Work out the finished part from the listing and answer in its coordinate system (mm). Face numbers are marked on the shaded views. A direction names the side the tool comes from. Give positions to 0.01 mm unless a question says otherwise; leave off trailing zeros. Loops run counter-clockwise (first coordinate to the right, second up) from the corner with the lowest first, then second, coordinate; pieces in that order, holes last. Notation, with made-up numbers: M 76,-16 L 87,-16 A28 cw 87,5 Z; hole C 83.5,63.5 d8. An arc over 180 degrees is marked long. Answer as a JSON object with one key per item and string values. Group by question number.
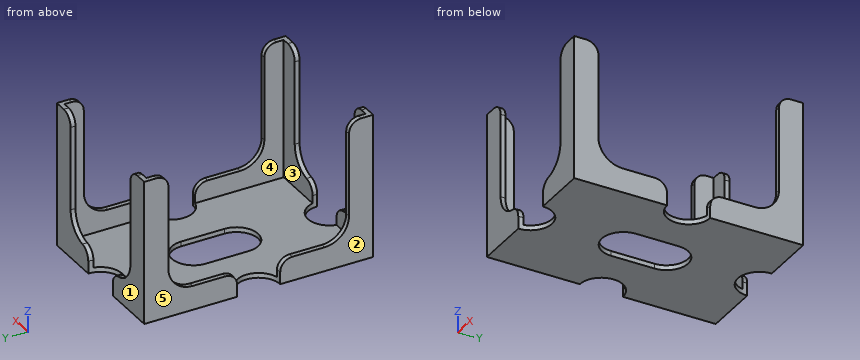
```python
from build123d import *

# Parameters (mm, degrees)
SKETCH008_W          = 50.7
SKETCH008_H          = 75.7
PAD002_DEPTH         = 47.6
THICKNESS002_T       = -1.6
POCKET004_DEPTH      = 37.851
POCKET004_DEPTH_BACK = 37.851
POCKET003_DEPTH      = 25.351
POCKET003_DEPTH_BACK = 25.351
SKETCH006_R          = 7.125
POCKET005_DEPTH      = 0.001
POCKET005_DEPTH_BACK = 47.601
FILLET001_R          = 4


with BuildPart() as part:
    # Sketch008 → Pad002 (new body)
    with BuildSketch(Plane.XY):
        Rectangle(SKETCH008_W, SKETCH008_H)
    extrude(amount=PAD002_DEPTH)

    # Thickness002
    thickness002_openings = [part.faces().sort_by_distance(p)[0] for p in [
        (0, 0, 47.6),
    ]]
    offset(amount=THICKNESS002_T, openings=thickness002_openings, kind=Kind.INTERSECTION)

    # Sketch007 → Pocket004 (cut, two sides)
    with BuildSketch(Plane.XZ) as pocket004_sk:
        with BuildLine():
            Line((-17.35, 47.6), (17.35, 47.6))
            Line((17.35, 47.6), (17.35, 16))
            ThreePointArc((9.35, 8), (15.006854, 10.343146), (17.35, 16))
            Line((9.35, 8), (-9.35, 8))
            ThreePointArc((-17.35, 16), (-15.006854, 10.343146), (-9.35, 8))
            Line((-17.35, 16), (-17.35, 47.6))
        make_face()
    extrude(amount=-POCKET004_DEPTH, mode=Mode.SUBTRACT)
    extrude(pocket004_sk.sketch, amount=POCKET004_DEPTH_BACK, mode=Mode.SUBTRACT)

    # Sketch005 → Pocket003 (cut, two sides)
    with BuildSketch(Plane.YZ) as pocket003_sk:
        with BuildLine():
            Line((-29.85, 47.6), (29.85, 47.6))
            Line((29.85, 47.6), (29.85, 16))
            ThreePointArc((21.85, 8), (27.506854, 10.343146), (29.85, 16))
            Line((21.85, 8), (-21.85, 8))
            ThreePointArc((-29.85, 16), (-27.506854, 10.343146), (-21.85, 8))
            Line((-29.85, 16), (-29.85, 47.6))
        make_face()
    extrude(amount=-POCKET003_DEPTH, mode=Mode.SUBTRACT)
    extrude(pocket003_sk.sketch, amount=POCKET003_DEPTH_BACK, mode=Mode.SUBTRACT)

    # Sketch006 → Pocket005 (cut, two sides)
    with BuildSketch(Plane.XY) as pocket005_sk:
        with Locations((0, 37.85)):
            Circle(SKETCH006_R)
        with Locations((0, -37.85)):
            Circle(SKETCH006_R)
        with Locations((25.35, 0)):
            Circle(SKETCH006_R)
        with Locations((-25.35, 0)):
            Circle(SKETCH006_R)
        with BuildLine():
            ThreePointArc((7.125, 7.125), (0, 14.25), (-7.125, 7.125))
            Line((-7.125, 7.125), (-7.125, -7.125))
            ThreePointArc((-7.125, -7.125), (0, -14.25), (7.125, -7.125))
            Line((7.125, 7.125), (7.125, -7.125))
        make_face()
    extrude(amount=-POCKET005_DEPTH, mode=Mode.SUBTRACT)
    extrude(pocket005_sk.sketch, amount=POCKET005_DEPTH_BACK, mode=Mode.SUBTRACT)

    # Fillet001
    fillet001_edges = [part.edges().sort_by_distance(p)[0] for p in [
        (24.544843, -7.079361, 8),
        (24.544843, 7.079361, 8),
        (24.55, 29.85, 47.6),
        (17.35, 37.05, 47.6),
        (7.079361, 37.044843, 8),
        (-7.079361, 37.044843, 8),
        (-17.35, 37.05, 47.6),
        (-24.55, 29.85, 47.6),
        (-24.544843, 7.079361, 8),
        (-24.544843, -7.079361, 8),
        (-24.55, -29.85, 47.6),
        (-17.35, -37.05, 47.6),
        (-7.079361, -37.044843, 8),
        (7.079361, -37.044843, 8),
        (17.35, -37.05, 47.6),
        (24.55, -29.85, 47.6),
    ]]
    fillet(fillet001_edges, radius=FILLET001_R)


solid = part.part
```
Item 1: A cutting plane is placed at D-D (y = 29). Determine the outline of the cut face in (x, z), and give its area (3 significant figures).
Item 2: A cutting plane is placed at B-B (x = 0). Determine the outline of the cut face in (y, z) (3 decimals), and give its area (3 significant figures).
Item 3: A cutting plane is placed at C-C (z = 29). Determine the outline of the cut face in (x, y), and give its area (3 significant figures).
Item 4: A cutting plane is placed at A-A (y = 0). Determine the outline of the cut face in (x, z) (3 decimals).
Item 5: Find the intervals of material crossed by probe 1 along Y at (x, z) = (19, 36); probe 2 along X at (y, z) = (-34, 20.5), in increasing order. Write a range as [from, to].
Item 6: For a pull along X with two mould halves and no side action, classify the marked faces 1, 2 and 3 as pulls with the +X half, pulls with the -X half, needs draft (parallel to the pull), parting line crosses it, or undercut.
Item 7: A tool of negligible diameter and unlimited length cuts with its end or side. For the marked faces 4 and 5, from which of +Z, -Z, +X, -X, +Y, -Y can it reach the whole face along a straight path? Write none if from no direction.
Item 8: Given pin 1 Ø1.8 at (x, y) = (-24.5, -17) entering from +Z; pin 2 Ø1.3 at (y, z) = (1.5, 1) entering from -X; pin 3 Ø4 at (x, y) = (-7.5, 26) entering from +Z; pin 4 Ø5 at (y, z) = (-26.5, 10) entering from +X, each flat-ended and moving along its own axis, determine where each tip first touches the part or whether it passes through.
The answers:
{
 "1": {"outline": "M -25.35,0 L 25.35,0 L 25.35,12.41 L 23.75,12.41 L 23.75,1.6 L -23.75,1.6 L -23.75,12.41 L -25.35,12.41 Z", "area": "116 mm^2"},
 "2": {"outline": "M -30.725,0 L -14.25,0 L -14.25,1.6 L -30.725,1.6 Z; M 14.25,0 L 30.725,0 L 30.725,1.6 L 14.25,1.6 Z", "area": "52.7 mm^2"},
 "3": {"outline": "M -25.35,-37.85 L -17.35,-37.85 L -17.35,-36.25 L -23.75,-36.25 L -23.75,-29.85 L -25.35,-29.85 Z; M -25.35,29.85 L -23.75,29.85 L -23.75,36.25 L -17.35,36.25 L -17.35,37.85 L -25.35,37.85 Z; M 17.35,-37.85 L 25.35,-37.85 L 25.35,-29.85 L 23.75,-29.85 L 23.75,-36.25 L 17.35,-36.25 Z; M 17.35,36.25 L 23.75,36.25 L 23.75,29.85 L 25.35,29.85 L 25.35,37.85 L 17.35,37.85 Z", "area": "92.2 mm^2"},
 "4": {"outline": "M -18.225,0 L -7.125,0 L -7.125,1.6 L -18.225,1.6 Z; M 7.125,0 L 18.225,0 L 18.225,1.6 L 7.125,1.6 Z"},
 "5": {"probe 1": "y = [-37.85, -36.25], [36.25, 37.85]", "probe 2": "x = [-25.35, -23.75], [23.75, 25.35]"},
 "6": {"face 1": "needs draft", "face 2": "pulls with the -X half", "face 3": "undercut"},
 "7": {"face 4": "+Z", "face 5": "+Z, -Z, -X, +Y, -Y"},
 "8": {"pin 1": "stops at z = 8", "pin 2": "stops at x = -18.56", "pin 3": "stops at z = 1.6", "pin 4": "stops at x = 25.35"}
}
